Check sheet for the modelled part. Datum: model origin and axes. Units: mm. Round coordinates to 2 decimals unless told otherwise and drop trailing zeros. Order: outer loops, then holes, each group sorted by start corner. A loop starts at its lowest first (then second) coordinate and runs counter-clockwise, first axis right, second up. Notation, with made-up numbers: (55, -37.5) -> (88, -37.5) arc R12 ccw to (88, -24.5) -> close; hole circle Ø2 at (-5.75, 46). An arc over 180 degrees is marked (long way). Answer in a Markdown table with one row per item.
```python
from build123d import *

# Parameters (mm, degrees)
BOSS_EXTRU_1_DEPTH           = 5
ENL_V_MAT_EXTRU_1_DEPTH      = 138.125803563
ENL_V_MAT_EXTRU_1_DEPTH_BACK = 138.125803563
ESQUISSE2_R                  = 3.5
ESQUISSE2_R_2                = 3
CONG_1_R                     = 5


with BuildPart() as part:
    # Esquisse1 → Boss.-Extru.1 (new body)
    with BuildSketch(Plane.XY):
        Polygon((0, 0), (0, 100), (-40, 100), (-93.693575035, 69), (-73.693575035, 34.358983849), (-40, 0), align=None)
    extrude(amount=BOSS_EXTRU_1_DEPTH)

    # Esquisse2 → Enlèv. mat.-Extru.1 (cut, two sides: drawn at the far end of the back side and taken through both)
    with BuildSketch(Plane.XY.offset(5).offset(-ENL_V_MAT_EXTRU_1_DEPTH_BACK)):
        with Locations((-20, 15)):
            Circle(ESQUISSE2_R)
        with Locations((-20, 50)):
            Circle(ESQUISSE2_R)
        with Locations((-20, 85)):
            Circle(ESQUISSE2_R)
        with Locations((-66.373066959, 61.679491924)):
            Circle(ESQUISSE2_R)
        with Locations((-85.497422612, 66.803847577)):
            Circle(ESQUISSE2_R_2)
        with Locations((-61.248711306, 80.803847577)):
            Circle(ESQUISSE2_R_2)
        with Locations((-47.248711306, 56.555136271)):
            Circle(ESQUISSE2_R_2)
        with Locations((-71.497422612, 42.555136271)):
            Circle(ESQUISSE2_R_2)
    extrude(amount=ENL_V_MAT_EXTRU_1_DEPTH + ENL_V_MAT_EXTRU_1_DEPTH_BACK, mode=Mode.SUBTRACT)

    # Congé1
    cong_1_edges = [part.edges().sort_by_distance(p)[0] for p in [
        (-40, 0, 2.5),
        (-73.693575035, 34.358983849, 2.5),
        (-93.693575035, 69, 2.5),
        (-40, 100, 2.5),
        (0, 100, 2.5),
        (0, 0, 2.5),
    ]]
    fillet(cong_1_edges, radius=CONG_1_R)


solid = part.part
```
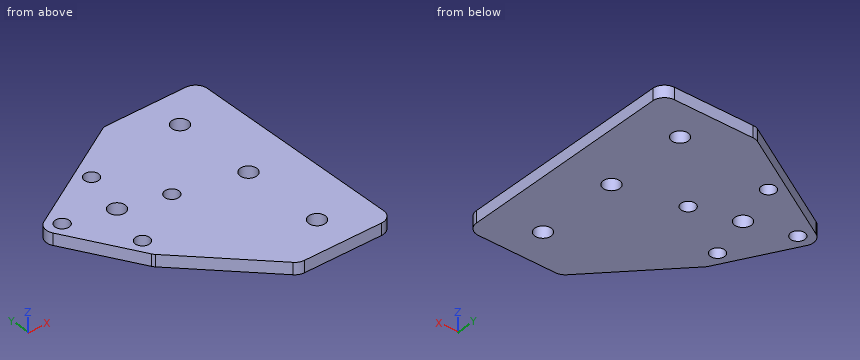
(1) Section check D-D on z = 3.35. Give the number of separate pieces and of enclosed holes in the cut face, plus the area to 3 significant figures.
Solutions:
| item | result |
|---|---|
| separate pieces | 1 |
| enclosed holes | 8 |
| area | 6,640 mm^2 |
(2) Section check B-B on y = 50. Record the boundary of the cut face in (x, z).
Solutions:
| item | result |
|---|---|
| outline | (-82.72, 0) -> (-23.5, 0) -> (-23.5, 5) -> (-82.72, 5) -> close; (-16.5, 0) -> (0, 0) -> (0, 5) -> (-16.5, 5) -> close |
(3) Scan lines: probe 1 along Y at (x, z) = (-20, 2.85); probe 2 along X at (y, z) = (44, 2.85); probe 3 along X at (y, z) = (63, 4.85). Record each from-to range of solid material in increasing order. Write a range as from..to.
Solutions:
| item | result |
|---|---|
| probe 1 | 0..11.5, 18.5..46.5, 53.5..81.5, 88.5..100 |
| probe 2 | -79.26..-74.13, -68.87..0 |
| probe 3 | -90.23..-69.61, -63.13..0 |
(4) Depth check by flat-ended pin: pin 1 Ø3.5 at (x, y) = (-71.5, 42.56) entering from +Z; pin 2 Ø2 at (x, z) = (-74.5, 2.5) entering from +Y; pin 3 Ø1 at (y, z) = (37.5, 0.5) entering from -X. Enter the tip coordinate at first touch or a pass-through.
Solutions:
| item | result |
|---|---|
| pin 1 | through |
| pin 2 | y = 80.66 |
| pin 3 | x = -75.8 |
(5) Section check A-A on x = -20. Record the boundary of the cut face in (y, z).
Solutions:
| item | result |
|---|---|
| outline | (0, 0) -> (11.5, 0) -> (11.5, 5) -> (0, 5) -> close; (18.5, 0) -> (46.5, 0) -> (46.5, 5) -> (18.5, 5) -> close; (53.5, 0) -> (81.5, 0) -> (81.5, 5) -> (53.5, 5) -> close; (88.5, 0) -> (100, 0) -> (100, 5) -> (88.5, 5) -> close |
(6) Section check C-C on x = -49. Record the boundary of the cut face in (y, z).
Solutions:
| item | result |
|---|---|
| outline | (9.18, 0) -> (54.12, 0) -> (54.12, 5) -> (9.18, 5) -> close; (58.99, 0) -> (94.8, 0) -> (94.8, 5) -> (58.99, 5) -> close |
